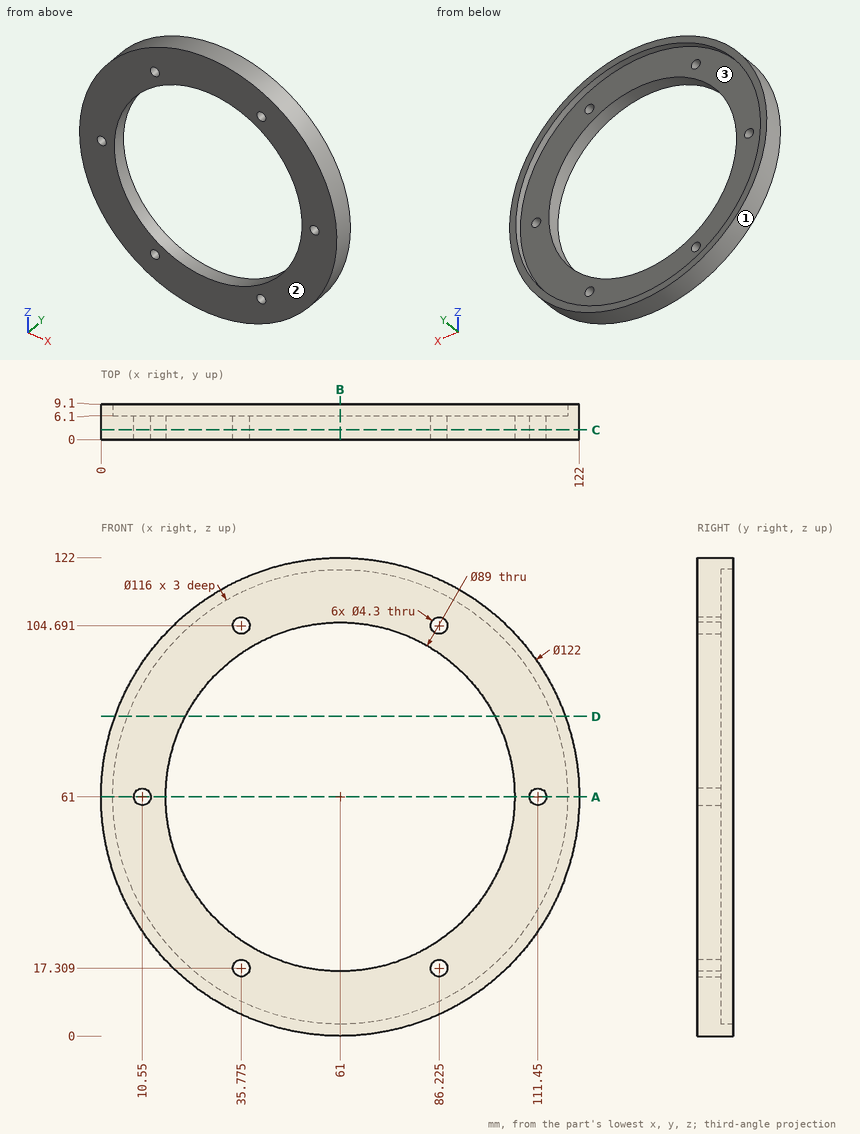
Job drawing, mm, ordinate dimensions from the low corner. One solid piece. Round coordinates to 2 decimals unless told otherwise and drop trailing zeros. Loops run counter-clockwise (first coordinate to the right, second up) from the corner with the lowest first, then second, coordinate; pieces in that order, holes last. Notation, with made-up numbers: M 49,-2.75 L 100,-2.75 A21 cw 100,12.25 Z; hole C -24,70 d8. An arc over 180 degrees is marked long. One line per question, with ' | ' between items. Start each with the question number.
Item 1: Two-plate mould, pull along X, no slides. Class the marked faces 1, 2 and 3: pulls with the +X half, pulls with the -X half, needs draft (parallel to the pull), parting line crosses it, or undercut.
Item 2: Pin check, flat tips, straight feed: pin 1 Ø5 at (x, y) = (65.5, 4.5) entering from +Z; pin 2 Ø3 at (x, y) = (33.5, 6.5) entering from -Z; pin 3 Ø2.5 at (x, z) = (86.22, 17.31) entering from -Y; pin 4 Ø2 at (y, z) = (6, 61.5) entering from +X. Stop position of each tip, or through.
Item 3: Cut at A-A, the plane z = 61. Write the cut outline in (x, y).
Item 4: Cut at B-B, the plane x = 61. Write the cut outline in (y, z), plus the area to 3 significant figures.
Item 5: Wall check: line 1 (X direction, y = 1.75, z = 61); line 2 (X direction, y = 7.15, z = 61); line 3 (X direction, y = 3, z = 62.5). Give the ranges that are in metal, low to high.
Item 6: Cut at C-C, the plane y = 2.5. Write the cut outline in (x, z) (3 decimals), plus the area to 3 significant figures.
Item 7: Cut at D-D, the plane z = 81.5. Write the cut outline in (x, y), plus the area to 3 significant figures.
Responses:
1) face 1: parting line crosses it | face 2: needs draft | face 3: undercut
2) pin 1: stops at z = 121.97 | pin 2: stops at z = 5.82 | pin 3: passes through | pin 4: stops at x = 122
3) outline: M 0,0 L 8.4,0 L 8.4,6.1 L 3,6.1 L 3,9.1 L 0,9.1 Z; M 12.7,0 L 16.5,0 L 16.5,6.1 L 12.7,6.1 Z; M 105.5,0 L 109.3,0 L 109.3,6.1 L 105.5,6.1 Z; M 113.6,0 L 122,0 L 122,9.1 L 119,9.1 L 119,6.1 L 113.6,6.1 Z
4) outline: M 0,0 L 9.1,0 L 9.1,3 L 6.1,3 L 6.1,16.5 L 0,16.5 Z; M 0,105.5 L 6.1,105.5 L 6.1,119 L 9.1,119 L 9.1,122 L 0,122 Z | area: 219 mm²
5) line 1: x = 0 to 8.4, 12.7 to 16.5, 105.5 to 109.3, 113.6 to 122 | line 2: x = 0 to 3, 119 to 122 | line 3: x = 0.02 to 9.01, 12.09 to 16.53, 105.47 to 109.91, 112.99 to 121.98
6) outline: C 61,61 d122; hole C 10.55,61 d4.3; hole C 61,61 d89; hole C 35.775,17.309 d4.3; hole C 35.775,104.691 d4.3; hole C 86.225,17.309 d4.3; hole C 86.225,104.691 d4.3; hole C 111.45,61 d4.3 | area: 5,380 mm²
7) outline: M 3.55,0 L 21.5,0 L 21.5,6.1 L 6.74,6.1 L 6.74,9.1 L 3.55,9.1 Z; M 100.5,0 L 118.45,0 L 118.45,9.1 L 115.26,9.1 L 115.26,6.1 L 100.5,6.1 Z | area: 238 mm²
